from build123d import *

# Parameters (mm, degrees)
F0_W     = 8
F0_H     = 12
F0_W_2   = 4
F0_H_2   = 8
F1_DEPTH = 2
F2_SIZE  = 0.4


with BuildPart() as f1:
    # F0 (on Top) → F1 (new body)
    with BuildSketch(Plane.XY):
        with Locations((-10.329974, -29.385177)):
            Rectangle(F0_W, F0_H)
        with Locations((-10.329974, -29.385177)):
            Rectangle(F0_W_2, F0_H_2, mode=Mode.SUBTRACT)
    extrude(amount=F1_DEPTH)

    # F2
    f2_edges = [f1.edges().sort_by_distance(p)[0] for p in [
        (-8.329974, -29.385177, 2),
        (-10.329974, -33.385177, 2),
        (-12.329974, -29.385177, 2),
        (-10.329974, -25.385177, 2),
        (-10.329974, -35.385177, 2),
        (-14.329974, -29.385177, 2),
        (-14.329974, -35.385177, 1),
        (-6.329974, -35.385177, 1),
        (-6.329974, -29.385177, 2),
        (-10.329974, -23.385177, 2),
        (-6.329974, -23.385177, 1),
        (-14.329974, -23.385177, 1),
        (-14.329974, -29.385177, 0),
        (-12.329974, -29.385177, 0),
        (-10.329974, -25.385177, 0),
        (-10.329974, -23.385177, 0),
        (-6.329974, -29.385177, 0),
        (-8.329974, -29.385177, 0),
        (-10.329974, -33.385177, 0),
        (-10.329974, -35.385177, 0),
    ]]
    chamfer(f2_edges, length=F2_SIZE)


solid = f1.part
Model file for the job. Use its own axes, mm. A direction names the side the tool comes from. Give positions to 0.01 mm unless a question says otherwise; leave off trailing zeros. Order: outer loops, then holes, each group sorted by start corner. A loop starts at its lowest first (then second) coordinate and runs counter-clockwise, first axis right, second up. Notation, with made-up numbers: M -17.75,39.5 L 30.25,39.5 A21 ccw 30.25,63.5 Z; hole C 75,57 d8. An arc over 180 degrees is marked long. Write item = value, one per line.
Q1. Cut at C-C, the plane x = -12. List the corners of the cut face in (y, z), then the cut area to 3 significant figures.
Derived:
outline = M -35.39,0.4 L -34.99,0 L -33.79,0 L -33.39,0.4 L -33.39,1.6 L -33.79,2 L -34.99,2 L -35.39,1.6 Z; M -25.39,0.4 L -24.99,0 L -23.79,0 L -23.39,0.4 L -23.39,1.6 L -23.79,2 L -24.99,2 L -25.39,1.6 Z
area = 7.36 mm2
Q2. Drill centre lines: line 1 (Y direction, x = -10.75, z = 1.1); line 2 (X direction, y = -27.75, z = 1.35); line 3 (X direction, y = -32.5, z = 0.3). Where is each one in solid material? Low to high. Write a range as [from, to].
Derived:
line_1 = [-35.39, -33.39], [-25.39, -23.39]
line_2 = [-14.33, -12.33], [-8.33, -6.33]
line_3 = [-14.23, -12.43], [-8.23, -6.43]
Q3. Tool access for faces 1 (the flat face through (-12.33, -29, 1)), 2 (the flat face through (-14.33, -29, 1)): list every direction of +Z, -Z, +X, -X, +Y, -Y with a clear straight run to the whole face (end or side of a thin tool).
Derived:
face_1 = +Z, -Z
face_2 = +Z, -Z, -X, +Y, -Y
Q4. Two-plate mould, pull along Y, no slides. Class faces 3 (the flat face through (-10, -25.385, 1)), 4 (the flat face through (-10, -35.385, 1)), 5 (the flat face through (-13, -29, 0)), 6 (the flat face through (-10, -33.385, 1)): pulls with the +Y half, pulls with the -Y half, needs draft (parallel to the pull), parting line crosses it, or undercut.
Derived:
face_3 = undercut
face_4 = pulls with the -Y half
face_5 = needs draft
face_6 = undercut
Q5. Cut at B-B, the plane z = 1.25. List the corners of the cut face in (x, y).
Derived:
outline = M -14.33,-34.99 L -13.93,-35.39 L -6.73,-35.39 L -6.33,-34.99 L -6.33,-23.79 L -6.73,-23.39 L -13.93,-23.39 L -14.33,-23.79 Z; hole M -12.33,-33.39 L -8.33,-33.39 L -8.33,-25.39 L -12.33,-25.39 Z
Q6. Cut at A-A, the plane y = -28.5. List the corners of the cut face in (x, z).
Derived:
outline = M -14.33,0.4 L -13.93,0 L -12.73,0 L -12.33,0.4 L -12.33,1.6 L -12.73,2 L -13.93,2 L -14.33,1.6 Z; M -8.33,0.4 L -7.93,0 L -6.73,0 L -6.33,0.4 L -6.33,1.6 L -6.73,2 L -7.93,2 L -8.33,1.6 Z
Q7. Cut at D-D, the plane y = -34.5. List the corners of the cut face in (x, z), then the cut area to 3 significant figures.
Derived:
outline = M -14.33,0.4 L -13.93,0 L -6.73,0 L -6.33,0.4 L -6.33,1.6 L -6.73,2 L -13.93,2 L -14.33,1.6 Z
area = 15.7 mm2
Q8. Flat gauge pins, fed straight in: pin 1 (2 mm diameter, centred on x = -9.5, y = -27.5, fed in from +Z); pin 2 (3 mm diameter, centred on x = -9.5, y = -32, fed in from +Z). Where does each tip first touch, or does it go through?
Derived:
pin_1 = through
pin_2 = 1.93
